Study the drawing (mm; zero at the part's minimum x, y, z) and answer. A direction names the side the tool comes from. Coordinates: 2 decimals unless noted, no trailing zeros. Order: outer loops, then holes, each group sorted by start corner. A loop starts at its lowest first (then second) coordinate and runs counter-clockwise, first axis right, second up. Notation, with made-up numbers: M 76.5,-4.75 L 117.5,-4.75 A25 cw 117.5,26.25 Z; hole C -26,-9.75 d6. An arc over 180 degrees is marked long. Use a Markdown table: item, result. Add a question column.
1) Find section C-C on y = 12.5. Write down the section's boundary in (x, z), plus the area to 3 significant figures.
2) Find the intervals of material crossed by probe 1 along Y at (x, z) = (23.4, 12.5), in increasing order. Write a range as [from, to].
3) The mould has two halves that part along Y. Classify the marked faces 1, 2 and 3: released by +Y, released by -Y, zero draft, split by the parting line, or undercut.
4) Find section D-D on x = 21. Write down the section's boundary in (y, z).
5) Find section A-A on x = 12.5. Write down the section's boundary in (y, z), plus the area to 3 significant figures.
6) For the marked faces 4 and 5, determine the directions among +Z, -Z, +X, -X, +Y, -Y from which every point of the face is accessible in a straight line to the end or side of a thin tool.
7) Find section B-B on z = 12.5. Write down the section's boundary in (x, y), plus the area to 3 significant figures.
8) Each of these flat-tipped pins is pushed along its axis until it touches: pin 1 Ø1 at (x, z) = (6.5, 18.5) entering from +Y; pin 2 Ø12 at (x, z) = (18, 4) entering from +Y; pin 3 Ø6.5 at (y, z) = (18.5, 6.5) entering from -X. Where does it stop, or does it pass through?
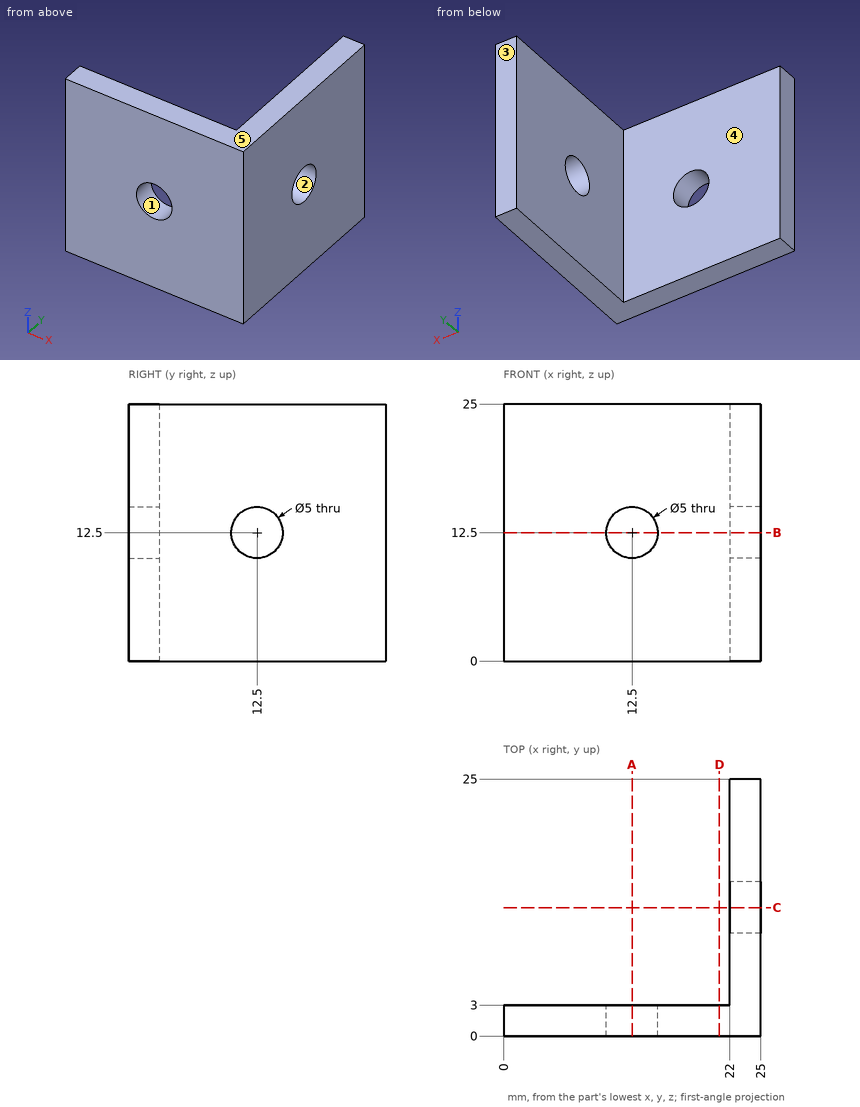
Check result:
| question | item | result |
|---|---|---|
| 1 | outline | M 22,0 L 25,0 L 25,10 L 22,10 Z; M 22,15 L 25,15 L 25,25 L 22,25 Z |
| 1 | area | 60.0 mm2 |
| 2 | probe 1 | y = [0, 10], [15, 25] |
| 3 | face 1 | zero draft |
| 3 | face 2 | undercut |
| 3 | face 3 | released by +Y |
| 4 | outline | M 0,0 L 3,0 L 3,25 L 0,25 Z |
| 5 | outline | M 0,0 L 3,0 L 3,10 L 0,10 Z; M 0,15 L 3,15 L 3,25 L 0,25 Z |
| 5 | area | 60.0 mm2 |
| 6 | face 4 | +Z, -Z, -X, +Y |
| 6 | face 5 | +Z, +X, -X, +Y, -Y |
| 7 | outline | M 0,0 L 10,0 L 10,3 L 0,3 Z; M 15,0 L 25,0 L 25,10 L 22,10 L 22,3 L 15,3 Z; M 22,15 L 25,15 L 25,25 L 22,25 Z |
| 7 | area | 111 mm2 |
| 8 | pin 1 | stops at y = 3 |
| 8 | pin 2 | stops at y = 25 |
| 8 | pin 3 | stops at x = 22 |
